from build123d import *

# Parameters (mm, degrees)
SKETCH2_W                = 10.16
SKETCH2_H                = 4.572
BASE_EXTRUDE_DEPTH       = 14.732
CUT_EXTRUDE1_DEPTH       = 1
CUT_EXTRUDE1_DEPTH_BACK  = 11.16
SKETCH4_R                = 1.905
CUT_EXTRUDE2_DEPTH       = 14.732
CUT_EXTRUDE4_DEPTH       = 0.0254
CUT_EXTRUDE5_DEPTH       = 0.0254
CUT_EXTRUDE6_DEPTH       = 0.0254
CUT_EXTRUDE7_DEPTH       = 2.54
SKETCH9_W                = 1.27
SKETCH9_H                = 7.62
BOSS_EXTRUDE_THIN1_DEPTH = 0.254
CUT_EXTRUDE8_DEPTH       = 1.27
LPATTERN1_COUNT          = 3
LPATTERN1_PITCH          = 2.54


with BuildPart() as part:
    # Sketch2 → Base-Extrude (new body)
    with BuildSketch(Plane(origin=(0, 3.81, 0), x_dir=(-1, 0, 0), z_dir=(0, 1, 0))):
        with Locations((-2.54, -0.889)):
            Rectangle(SKETCH2_W, SKETCH2_H)
    extrude(amount=BASE_EXTRUDE_DEPTH)

    # Sketch3 → Cut-Extrude1 (cut, two sides)
    with BuildSketch(Plane.ZY.offset(2.54)) as cut_extrude1_sk:
        Polygon((-1.905, 18.542), (-1.905, 12.446), (1.397, 11.938), (1.397, 18.542), align=None)
    extrude(amount=CUT_EXTRUDE1_DEPTH, mode=Mode.SUBTRACT)
    extrude(cut_extrude1_sk.sketch, amount=-CUT_EXTRUDE1_DEPTH_BACK, mode=Mode.SUBTRACT)

    # Sketch4 → Cut-Extrude2 (cut)
    with BuildSketch(Plane.XY.offset(-1.905)):
        with Locations((2.54, 15.875)):
            Circle(SKETCH4_R)
    extrude(amount=-CUT_EXTRUDE2_DEPTH, mode=Mode.SUBTRACT)

    # Sketch5 → Cut-Extrude4 (cut)
    with BuildSketch(Plane.ZY.offset(2.54)):
        Polygon((-3.175, 12.641384615), (1.397, 11.938), (1.397, 3.81), (-3.175, 3.81), align=None)
    extrude(amount=-CUT_EXTRUDE4_DEPTH, mode=Mode.SUBTRACT)

    # Sketch6 → Cut-Extrude5 (cut)
    with BuildSketch(Plane(origin=(7.62, 0, 0), x_dir=(0, 0, -1), z_dir=(1, 0, 0))):
        Polygon((-1.397, 11.938), (3.175, 12.641384615), (3.175, 3.81), (-1.397, 3.81), align=None)
    extrude(amount=-CUT_EXTRUDE5_DEPTH, mode=Mode.SUBTRACT)

    # Sketch7 → Cut-Extrude6 (cut)
    with BuildSketch(Plane(origin=(0, 0, -3.175), x_dir=(-1, 0, 0), z_dir=(0, 0, -1))):
        Polygon((-7.62, 18.542), (-7.62, 12.641384615), (-6.35, 12.641384615), (-6.35, 7.112), (1.27, 7.112), (1.27, 12.641384615), (2.54, 12.641384615), (2.54, 18.542), align=None)
    extrude(amount=-CUT_EXTRUDE6_DEPTH, mode=Mode.SUBTRACT)

    # Sketch8 → Cut-Extrude7 (cut)
    with BuildSketch(Plane.XY.offset(-1.905)):
        with BuildLine():
            Line((7.62, 16.764), (7.62, 17.78))
            ThreePointArc((7.62, 17.78), (7.112, 17.272), (7.62, 16.764))
        make_face()
        with BuildLine():
            Line((-2.54, 16.764), (-2.54, 17.78))
            ThreePointArc((-2.54, 17.78), (-2.032, 17.272), (-2.54, 16.764))
        make_face()
    extrude(amount=-CUT_EXTRUDE7_DEPTH, mode=Mode.SUBTRACT)

    # Sketch9 → Boss-Extrude-Thin1 (add, symmetric)
    with BuildSketch(Plane.XY):
        Rectangle(SKETCH9_W, SKETCH9_H)
    boss_extrude_thin1 = extrude(amount=BOSS_EXTRUDE_THIN1_DEPTH, both=True)

    # Sketch11 → Cut-Extrude8 (cut)
    with BuildSketch(Plane.XY.offset(0.254)):
        Polygon((0.635, 0.508), (0.635, -3.81), (0.381, -3.81), (0.381, 0), align=None)
        Polygon((-0.635, 0.508), (-0.635, -3.81), (-0.381, -3.81), (-0.381, 0), align=None)
    cut_extrude8 = extrude(amount=-CUT_EXTRUDE8_DEPTH, mode=Mode.SUBTRACT)

    # LPattern1: Boss-Extrude-Thin1, Cut-Extrude8 ×3
    with Locations(*[(i * LPATTERN1_PITCH, 0, 0) for i in range(1, LPATTERN1_COUNT)]):
        add(boss_extrude_thin1)
        add(cut_extrude8, mode=Mode.SUBTRACT)


solid = part.part
Here's how the part is built. I have some questions about the finished solid (model axes, mm). A direction names the side the tool comes from. Coordinates: 2 decimals unless noted, no trailing zeros. Order: outer loops, then holes, each group sorted by start corner. A loop starts at its lowest first (then second) coordinate and runs counter-clockwise, first axis right, second up. Notation, with made-up numbers: M 22,16 L 31,16 A31 ccw 31,44 Z; hole C 38,-38.75 d3. An arc over 180 degrees is marked long. Answer as CSV lines item,"result".
Item 1: On a 3-axis mill with a long thin cutter (end or side, diameter ignored), from which of +Z, -Z, +X, -X, +Y, -Y can I reach the whole of each face in a straight line? I mean faces 4 (the face through (3, 1, 0.254)), 5 (the face through (1, 14, -1.905)), 6 (the face through (0, 1, -0.254)). Say none if no direction works.
Results found:
face 4,"+Z, +X, -X, -Y"
face 5,"+Z, +X, -X, +Y"
face 6,"-Z, +X, -X, -Y"
Item 2: Imagine slicing it at A-A on y = 2.75. Write out the boundary of the cut face in (x, z) (3 decimals).
Results found:
outline,"M -0.635,-0.254 L 0.635,-0.254 L 0.635,0.254 L -0.635,0.254 Z; M 1.905,-0.254 L 3.175,-0.254 L 3.175,0.254 L 1.905,0.254 Z; M 4.445,-0.254 L 5.715,-0.254 L 5.715,0.254 L 4.445,0.254 Z"
Item 3: We'd pull the mould along X, two halves only. Please class faces 1 (the face through (0, 1, 0.254)), 2 (the face through (7.595, 8, -1)), 3 (the face through (3, 13, -3.15)): +X half, -X half, draft (parallel to the pull), parting line (faces both ways), or undercut.
Results found:
face 1,"draft"
face 2,"+X half"
face 3,"undercut"
Item 4: Imagine slicing it at B-B on x = 2.54. Write out the boundary of the cut face in (y, z) (3 decimals).
Results found:
outline,"M -3.81,-0.254 L 3.81,-0.254 L 3.81,-3.175 L 7.112,-3.175 L 7.112,-3.15 L 13.97,-3.15 L 13.97,-1.905 L 12.446,-1.905 L 11.938,1.397 L 3.81,1.397 L 3.81,0.254 L -3.81,0.254 Z; M 17.78,-3.15 L 18.542,-3.15 L 18.542,-1.905 L 17.78,-1.905 Z"
Item 5: If I drill on line 1 (X direction, y = 3.5, z = 0.2) (3 decimals); line 2 (Y direction, x = 2.54, z = -2.6); line 3 (X direction, y = 9.75, z = 0.75), over which ranges is the centre line in solid material (lowest first)?
Results found:
line 1,"-0.635 to 0.635, 1.905 to 3.175, 4.445 to 5.715"
line 2,"3.81 to 13.97, 17.78 to 18.54"
line 3,"-2.51 to 7.59"
Item 6: For pin 1 (3 mm diameter, centred on x = 4, y = 12, fed in from -Z); pin 2 (3 mm diameter, centred on x = 0, y = 16.5, fed in from +Z) (3 decimals); pin 3 (5 mm diameter, centred on x = 3.5, y = 0, fed in from -Z); pin 4 (1.5 mm diameter, centred on y = 14.5, z = -1, fed in from -X), each with a flat end and sliding along its axis, tell me the tip position at first contact or that it passes through.
Results found:
pin 1,"z = -3.15"
pin 2,"z = -1.905"
pin 3,"z = -0.25"
pin 4,"through"
Item 7: Imagine slicing it at D-D on z = -2.5. Write out the boundary of the cut face in (x, y) (3 decimals).
Results found:
outline,"M -2.54,12.538 L -2.515,12.538 L -2.515,3.81 L 7.595,3.81 L 7.595,12.538 L 7.62,12.538 L 7.62,16.764 A0.508 cw 7.62,17.78 L 7.62,18.542 L -2.54,18.542 L -2.54,17.78 A0.508 cw -2.54,16.764 Z; hole C 2.54,15.875 d3.81"
Item 8: Imagine slicing it at C-C on x = -1.5. Write out the boundary of the cut face in (y, z) (3 decimals).
Results found:
outline,"M 3.81,-3.175 L 12.641,-3.175 L 12.641,-3.15 L 18.542,-3.15 L 18.542,-1.905 L 12.446,-1.905 L 11.938,1.397 L 3.81,1.397 Z"
